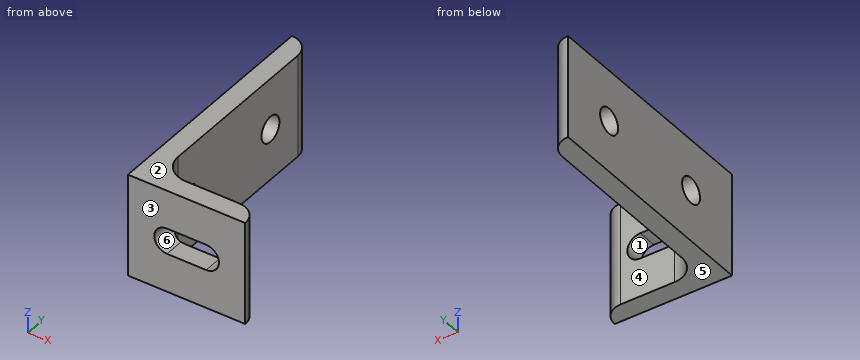
from build123d import *

# Parameters (mm, degrees)
BOSS_EXTRUDE1_DEPTH = 16.6624
FILLET1_R           = 6.35
CUT_EXTRUDE1_REACH  = 88.808
SKETCH3_R           = 4.1656
CUT_EXTRUDE2_REACH  = 88.808


with BuildPart() as part:
    # Sketch2 → Boss-Extrude1 (new, symmetric)
    with BuildSketch(Plane.XY):
        with BuildLine():
            Line((0, 0), (0, 76.2))
            Line((0, 76.2), (6.35, 76.2))
            Line((6.35, 76.2), (6.35, 14.2748))
            ThreePointArc((6.35, 14.2748), (8.67112018, 8.67112018), (14.2748, 6.35))
            Line((14.2748, 6.35), (38.1, 6.35))
            Line((38.1, 6.35), (38.1, 0))
            Line((38.1, 0), (0, 0))
        make_face()
    extrude(amount=BOSS_EXTRUDE1_DEPTH, both=True)

    # Fillet1
    fillet1_edges = [part.edges().sort_by_distance(p)[0] for p in [
        (38.1, 6.35, 0),
        (6.35, 76.2, 0),
    ]]
    fillet(fillet1_edges, radius=FILLET1_R - 0.0001)  # a hair under: the kernel refuses the full size

    # Sketch3 → Cut-Extrude1 (cut, up to next)
    with BuildSketch(Plane.ZY, mode=Mode.PRIVATE) as cut_extrude1_sk1:
        with Locations(Location((0, 57.15, 0), (0, 0, 270))):
            Circle(SKETCH3_R)
    cut_extrude1_tool1 = extrude(cut_extrude1_sk1.sketch, amount=-CUT_EXTRUDE1_REACH, mode=Mode.PRIVATE) & part.part
    # Sketch3 → Cut-Extrude1 (cut, up to next)
    with BuildSketch(Plane.ZY, mode=Mode.PRIVATE) as cut_extrude1_sk2:
        with Locations(Location((0, 19.05, 0), (0, 0, 270))):
            Circle(SKETCH3_R)
    cut_extrude1_tool2 = extrude(cut_extrude1_sk2.sketch, amount=-CUT_EXTRUDE1_REACH, mode=Mode.PRIVATE) & part.part
    add(cut_extrude1_tool1.solids().sort_by_distance((0, 57.15, 0))[0], mode=Mode.SUBTRACT)
    add(cut_extrude1_tool2.solids().sort_by_distance((0, 19.05, 0))[0], mode=Mode.SUBTRACT)

    # Sketch4 → Cut-Extrude2 (cut, up to next)
    with BuildSketch(Plane.XZ, mode=Mode.PRIVATE) as cut_extrude2_sk1:
        with BuildLine():
            Line((25.4, 4.1656), (12.7, 4.1656))
            ThreePointArc((12.7, 4.1656), (8.5344, 0), (12.7, -4.1656))
            Line((12.7, -4.1656), (25.4, -4.1656))
            ThreePointArc((25.4, -4.1656), (29.5656, 0), (25.4, 4.1656))
        make_face()
    cut_extrude2_tool1 = extrude(cut_extrude2_sk1.sketch, amount=-CUT_EXTRUDE2_REACH, mode=Mode.PRIVATE) & part.part
    add(cut_extrude2_tool1.solids().sort_by_distance((19.05, 0, 0))[0], mode=Mode.SUBTRACT)


solid = part.part
Build history of the part. All positions in model axes, mm. Face numbers are marked on the shaded views. A direction names the side the tool comes from. Coordinates: 2 decimals unless noted, no trailing zeros. Order: outer loops, then holes, each group sorted by start corner. A loop starts at its lowest first (then second) coordinate and runs counter-clockwise, first axis right, second up. Notation, with made-up numbers: (8, 73) -> (27, 73) arc R37 cw to (27, 112) -> close; hole circle Ø9 at (28.5, 35). An arc over 180 degrees is marked (long way). One line per item, written item: value.
(1) Probe line 1 (X direction, y = 27, z = 4); line 2 (Z direction, x = 2.5, y = 57.15). List the from-to ranges inside material, lowest first. Write a range as [from, to].
Checked values:
line 1: [0, 6.35]
line 2: [-16.66, -4.17], [4.17, 16.66]
(2) Drop flat-ended pins along their axis: pin 1 Ø1 at (x, z) = (32.5, 12) entering from +Y; pin 2 Ø6.5 at (y, z) = (57.15, 0) entering from -X; pin 3 Ø19 at (x, z) = (22, 8) entering from +Y; pin 4 Ø4 at (y, z) = (39, -11.5) entering from +X. Give the stop position or say it passes through.
Checked values:
pin 1: y = 6.35
pin 2: through
pin 3: y = 6.55
pin 4: x = 6.35
(3) Slice it at C-C, the plane z = -2. Count the separate pieces of the cut face and the enclosed holes in it, plus the area to 3 significant figures.
Checked values:
separate pieces: 4
enclosed holes: 0
area: 459 mm2
(4) Tool access for the marked faces 4, 5 and 6: list every direction of +Z, -Z, +X, -X, +Y, -Y with a clear straight run to the whole face (end or side of a thin tool).
Checked values:
face 4: +Z, -Z, +X, +Y
face 5: -Z, +X, -X, +Y, -Y
face 6: +Y, -Y
(5) Mould opens along Z. For the marked faces 1, 2 and 3 say: pulls with the +Z half, pulls with the -Z half, needs draft (parallel to the pull), parting line crosses it, or undercut.
Checked values:
face 1: undercut
face 2: pulls with the +Z half
face 3: needs draft
(6) Slice it at A-A, the plane y = 57.15. List the corners of the cut face in (x, z).
Checked values:
outline: (0, -16.66) -> (6.35, -16.66) -> (6.35, -4.17) -> (0, -4.17) -> close; (0, 4.17) -> (6.35, 4.17) -> (6.35, 16.66) -> (0, 16.66) -> close
